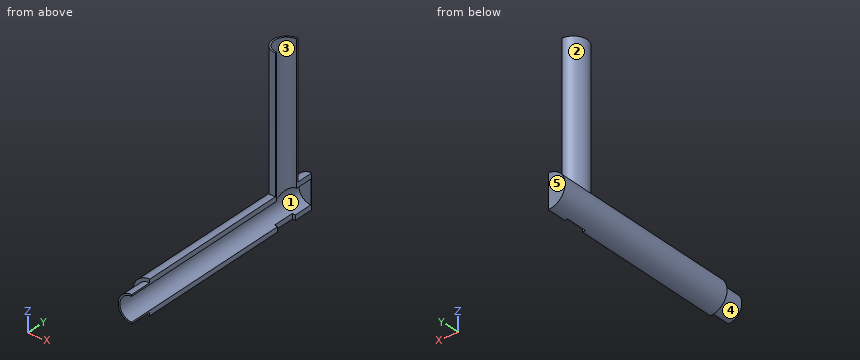
```python
from build123d import *

# Parameters (mm, degrees)
SKETCH1_W                = 15.3
SKETCH1_H                = 180
SKETCH1_W_2              = 12.3
SKETCH1_H_2              = 20
BOSS_EXTRUDE1_DEPTH      = 120
BOSS_EXTRUDE1_DEPTH_BACK = 9
SKETCH4_R                = 12.5
BOSS_EXTRUDE2_START      = -25
SKETCH6_W                = 40
SKETCH6_H                = 18
SKETCH6_W_2              = 36
SKETCH6_H_2              = 14
BOSS_EXTRUDE2_DEPTH      = 10
SKETCH2_R                = 10.8
CUT_EXTRUDE1_DEPTH       = 199
SKETCH5_R                = 11
CUT_EXTRUDE2_DEPTH       = 133
SKETCH7_W                = 36
SKETCH7_H                = 14
CUT_EXTRUDE3_DEPTH       = 15
BOSS_EXTRUDE3_START      = -11
SKETCH8_W                = 5.5
SKETCH8_H                = 22
BOSS_EXTRUDE3_DEPTH      = 6
SKETCH9_R                = 1.75
BOSS_EXTRUDE4_DEPTH      = 2
SKETCH10_W               = 36
SKETCH10_H               = 14
SKETCH10_R               = 4
BOSS_EXTRUDE5_DEPTH      = 1
CUT_EXTRUDE5_DEPTH       = 215


with BuildPart() as part:
    # Sketch1 → Revolve1 (revolve)
    with BuildSketch(Plane.XY, mode=Mode.PRIVATE) as revolve1_sk:
        with Locations((-7.65, 90)):
            Rectangle(SKETCH1_W, SKETCH1_H)
        with Locations((-6.15, -10)):
            Rectangle(SKETCH1_W_2, SKETCH1_H_2)
    revolve(revolve1_sk.sketch.rotate(Axis((0, 259.808396335, 0), (0, -1, 0)), 270), axis=Axis((0, 259.808396335, 0), (0, -1, 0)))

    # Sketch4 → Boss-Extrude1 (add, two sides: drawn at the far end of the back side and taken through both)
    with BuildSketch(Plane.XY.offset(15.3).offset(-BOSS_EXTRUDE1_DEPTH_BACK)):
        with Locations((0, 152.071263422)):
            Circle(SKETCH4_R)
    extrude(amount=BOSS_EXTRUDE1_DEPTH + BOSS_EXTRUDE1_DEPTH_BACK)

    # Sketch6 → Boss-Extrude2 (add)
    with BuildSketch(Plane.ZY.offset(12.5).offset(BOSS_EXTRUDE2_START)):
        with Locations((115.3, 152.071263422)):
            Rectangle(SKETCH6_W, SKETCH6_H)
        with Locations((115.3, 152.071263422)):
            Rectangle(SKETCH6_W_2, SKETCH6_H_2, mode=Mode.SUBTRACT)
    extrude(amount=BOSS_EXTRUDE2_DEPTH)

    # Sketch2 → Cut-Extrude1 (cut)
    with BuildSketch(Plane.XZ.offset(20)):
        with Locations(Location((0, 0, 0), (0, 0, 270))):
            Circle(SKETCH2_R)
    extrude(amount=-CUT_EXTRUDE1_DEPTH, mode=Mode.SUBTRACT)

    # Sketch5 → Cut-Extrude2 (cut)
    with BuildSketch(Plane.XY.offset(135.3)):
        with Locations((0, 152.071263422)):
            Circle(SKETCH5_R)
    extrude(amount=-CUT_EXTRUDE2_DEPTH, mode=Mode.SUBTRACT)

    # Sketch7 → Cut-Extrude3 (cut)
    with BuildSketch(Plane(origin=(12.5, 0, 0), x_dir=(0, 0, -1), z_dir=(1, 0, 0))):
        with Locations((-115.3, 152.071263422)):
            Rectangle(SKETCH7_W, SKETCH7_H)
    extrude(amount=-CUT_EXTRUDE3_DEPTH, mode=Mode.SUBTRACT)

    # Sketch8 → Boss-Extrude3 (add)
    with BuildSketch(Plane.XY.offset(97.3).offset(BOSS_EXTRUDE3_START)):
        with Locations((2.75, 152.071263422)):
            Rectangle(SKETCH8_W, SKETCH8_H)
        with BuildLine():
            ThreePointArc((8.485281374, 159.071263422), (7.105810702, 160.468135117), (5.5, 161.597542863))
            Line((5.5, 161.597542863), (5.5, 142.54498398))
            ThreePointArc((5.5, 142.54498398), (7.105810702, 143.674391726), (8.485281374, 145.071263422))
            ThreePointArc((8.485281374, 145.071263422), (11, 152.071263422), (8.485281374, 159.071263422))
        make_face()
    extrude(amount=-BOSS_EXTRUDE3_DEPTH)

    # Sketch9 → Boss-Extrude4 (add)
    with BuildSketch(Plane.ZY):
        with Locations((83.05, 159.671263422)):
            Circle(SKETCH9_R)
        with Locations(Location((83.05, 144.471263422, 0), (0, 0, 180))):
            Circle(SKETCH9_R)
    extrude(amount=BOSS_EXTRUDE4_DEPTH)

    # Sketch10 → Boss-Extrude5 (add)
    with BuildSketch(Plane(origin=(12.5, 0, 0), x_dir=(0, 0, -1), z_dir=(1, 0, 0))):
        with Locations((-115.3, 152.071263422)):
            Rectangle(SKETCH10_W, SKETCH10_H)
        with Locations((-127.3, 152.071263422)):
            Circle(SKETCH10_R, mode=Mode.SUBTRACT)
        with Locations((-115.3, 152.071263422)):
            Circle(SKETCH10_R, mode=Mode.SUBTRACT)
        with Locations((-103.3, 152.071263422)):
            Circle(SKETCH10_R, mode=Mode.SUBTRACT)
    extrude(amount=-BOSS_EXTRUDE5_DEPTH)

    # Sketch12 → Cut-Extrude5 (cut)
    with BuildSketch(Plane.XY.offset(135.3)):
        with BuildLine():
            Line((15.3, 180), (0, 180))
            Line((0, 180), (0, 164.571263422))
            ThreePointArc((0, 164.571263422), (4.677071733, 163.663286541), (8.674675786, 161.071263422))
            Line((8.674675786, 161.071263422), (12.5, 161.071263422))
            Line((12.5, 161.071263422), (12.5, 143.071263422))
            Line((12.5, 143.071263422), (8.674675786, 143.071263422))
            ThreePointArc((8.674675786, 143.071263422), (4.677071733, 140.479240302), (0, 139.571263422))
            Line((0, 139.571263422), (0, -20))
            Line((0, -20), (15.3, -20))
            Line((15.3, -20), (15.3, 180))
        make_face()
        with BuildLine():
            ThreePointArc((8.674675786, 161.071263422), (4.677071733, 163.663286541), (0, 164.571263422))
            Line((0, 164.571263422), (0, 163.071263422))
            ThreePointArc((0, 163.071263422), (7.778174593, 159.849438015), (11, 152.071263422))
            ThreePointArc((11, 152.071263422), (7.778174593, 144.293088829), (0, 141.071263422))
            Line((0, 141.071263422), (0, 139.571263422))
            ThreePointArc((0, 139.571263422), (4.677071733, 140.479240302), (8.674675786, 143.071263422))
            Line((8.674675786, 143.071263422), (12.5, 143.071263422))
            Line((12.5, 143.071263422), (12.5, 161.071263422))
            Line((12.5, 161.071263422), (8.674675786, 161.071263422))
        make_face()
        with BuildLine():
            ThreePointArc((11, 152.071263422), (7.778174593, 159.849438015), (0, 163.071263422))
            Line((0, 163.071263422), (0, 161.806579982))
            Line((0, 161.806579982), (-2.604703903, 161.806579982))
            Line((-2.604703903, 161.806579982), (-2.604703903, 142.047887239))
            Line((-2.604703903, 142.047887239), (0, 142.047887239))
            Line((0, 142.047887239), (0, 141.071263422))
            ThreePointArc((0, 141.071263422), (7.778174593, 144.293088829), (11, 152.071263422))
        make_face()
    extrude(amount=-CUT_EXTRUDE5_DEPTH, mode=Mode.SUBTRACT)


solid = part.part
```
The model under review builds one solid part; all positions refer to its coordinate system, in mm. Face numbers are marked on the shaded views. A direction names the side the tool comes from. Coordinates: 2 decimals unless noted, no trailing zeros. Order: outer loops, then holes, each group sorted by start corner. A loop starts at its lowest first (then second) coordinate and runs counter-clockwise, first axis right, second up. Notation, with made-up numbers: (64, 21.5) -> (97, 21.5) arc R18 cw to (97, 47.5) -> close; hole circle Ø2 at (34, 7.25). An arc over 180 degrees is marked (long way). Answer in a Markdown table with one row per item. Add a question column.
Item 1: We need section A-A on z = 0. Write out the cut boundary in (x, y), plus the area to 3 significant figures.
Item 2: Clearance check with flat-ended pins moving along their axes: pin 1 (0.8 mm diameter, centred on x = -0.5, z = -13.5, fed in from -Y); pin 2 (4 mm diameter, centred on x = -10.5, z = 25.5, fed in from +Y); pin 3 (1 mm diameter, centred on x = -9, y = 123, fed in from -Z). State where each tip first meets the part, or that it passes through.
Item 3: We need section C-C on z = 35. Write out the cut boundary in (x, y), plus the area to 3 significant figures.
Item 4: Machinability: for the marked faces 4 and 5, which of the approach directions +Z, -Z, +X, -X, +Y, -Y give a long, thin tool a straight path to every point of the face, cutting with its end or side? Answer none if there is none.
Item 5: We need section B-B on y = 31.5. Write out the cut boundary in (x, z).
Item 6: Mouldability with a two-part tool opening along Y and no side actions: class the marked faces 1, 2 and 3 as +Y half, -Y half, draft (parallel to the pull), parting line (faces both ways), or undercut.
Item 7: To check wall thickness, follow probe 1 along Z at (x, y) = (-1, 86.5); probe 2 along Z at (x, y) = (-2.75, -5); probe 3 along X at (y, z) = (75, -1). State the ranges of each line that lie inside material, in increasing order.
Final values:
| question | item | result |
|---|---|---|
| 1 | outline | (-15.3, 0) -> (-12.3, 0) -> (-12.3, -20) -> (-10.8, -20) -> (-10.8, 179) -> (0, 179) -> (0, 180) -> (-15.3, 180) -> close |
| 1 | area | 851 mm2 |
| 2 | pin 1 | stops at y = 0 |
| 2 | pin 2 | stops at y = 161.24 |
| 2 | pin 3 | stops at z = -12.72 |
| 3 | outline | (0, 139.57) -> (0, 141.07) arc R11 cw to (0, 163.07) -> (0, 164.57) arc R12.5 ccw to start |
| 3 | area | 55.4 mm2 |
| 4 | face 4 | -X, -Y |
| 4 | face 5 | +Z, -Z, +X, -X, +Y |
| 5 | outline | (0, -15.3) -> (0, -10.8) arc R10.8 cw to (0, 10.8) -> (0, 15.3) arc R15.3 ccw to start |
| 6 | face 1 | draft |
| 6 | face 2 | parting line |
| 6 | face 3 | undercut |
| 7 | probe 1 | z = -15.27 to -10.75, 10.75 to 15.27 |
| 7 | probe 2 | z = -11.99 to -10.44, 10.44 to 11.99 |
| 7 | probe 3 | x = -15.27 to -10.75 |
